Can you work these out from the drawing? Everything is in mm from the part's minimum corner. Give positions to 0.01 mm unless a question says otherwise; leave off trailing zeros. Loops run counter-clockwise (first coordinate to the right, second up) from the corner with the lowest first, then second, coordinate; pieces in that order, holes last.
Q1. Will these pins go through, and if not, where does the flat tip stop? P1, Ø3.5, axis at x = 54.5, y = 5, coming from the -Z side; P2, Ø5, axis at x = 10.5, y = 5, coming from the -Z side.
Q2. If we section it at B-B (x = 32.5): Please give me the cut outline in (y, z), plus the area to 3 significant figures.
Q3. I need wall thicknesses on line 1 (Y direction, x = 10.5, z = 8.75); line 2 (Z direction, x = 32.5, y = 6.75); line 3 (X direction, y = 6, z = 7). Which ranges of each line are inside material? Lowest first, please.
Q4. If we section it at A-A (z = 38): Please give me the cut outline in (x, y), plus the area to 3 significant figures.
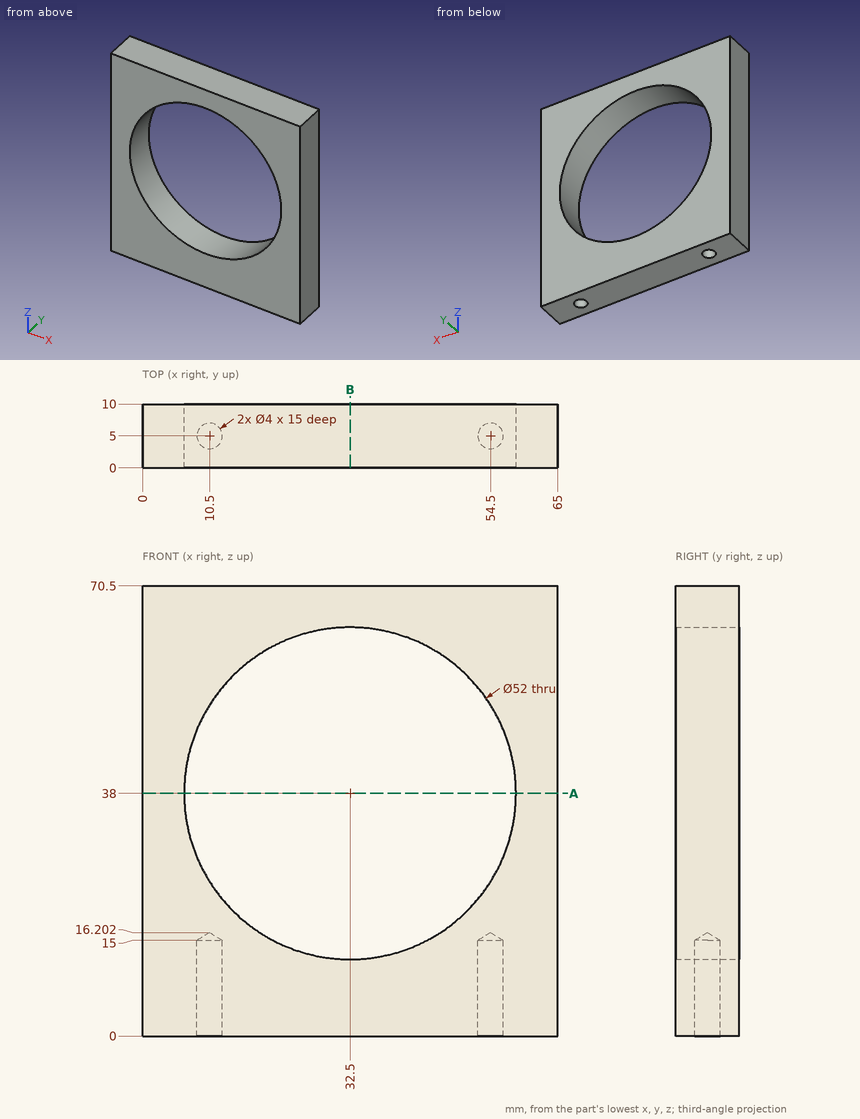
Check sheet entries:
1. P1: stops at z = 15.15
1. P2: stops at z = 0
2. outline: (0, 0) - (10, 0) - (10, 12) - (0, 12) - close; (0, 64) - (10, 64) - (10, 70.5) - (0, 70.5) - close
2. area: 185 mm2
3. line 1: y = 0 to 3, 7 to 10
3. line 2: z = 0 to 12, 64 to 70.5
3. line 3: x = 0 to 8.77, 12.23 to 52.77, 56.23 to 65
4. outline: (0, 0) - (6.5, 0) - (6.5, 10) - (0, 10) - close; (58.5, 0) - (65, 0) - (65, 10) - (58.5, 10) - close
4. area: 130 mm2
